Design review of the part built by this model. Coordinates are the model's own, in mm. Face numbers are marked on the shaded views. A direction names the side the tool comes from. Give positions to 0.01 mm unless a question says otherwise; leave off trailing zeros. Loops run counter-clockwise (first coordinate to the right, second up) from the corner with the lowest first, then second, coordinate; pieces in that order, holes last. Notation, with made-up numbers: (64, 7) - (82, 7) arc R26 cw to (82, 31) - close; hole circle Ø10 at (79.25, 67.5). An arc over 180 degrees is marked (long way). Write each question's results on one line, items separated by ' | '.
Autodesk Inventor part; units mm, degrees
ref_plane "YZ Plane" through (0, 0, 0) normal (1, 0, 0) x (0, 1, 0)
ref_plane "XZ Plane" through (0, 0, 0) normal (0, 1, 0) x (-1, 0, 0)
ref_plane "XY Plane" through (0, 0, 0) normal (0, 0, 1) x (1, 0, 0)
sketch "Sketch1" plane through (0, 0, 0) normal (0, 1, 0) x (-1, 0, 0)
  line L0 (-54.2742, 0) -> (84.3226, 0) construction
  line L1 (-6.35, -36.068) -> (57.15, -36.068)
  line L2 (57.15, -36.068) -> (57.15, 36.068)
  line L3 (57.15, 36.068) -> (-6.35, 36.068)
  line L4 (-31.75, 10.668) -> (-31.75, -10.668)
  circle A0 centre (0, 0) radius 17 construction
  circle A1 centre (0, 0) radius 20.81
  line L5 (0, 0) -> (-18.9066, 32.7472) construction
  circle A2 centre (0, 0) radius 3.81 construction
  arc A3 (-6.35, 36.068) -> (-31.75, 10.668) centre (-6.35, 10.668) ccw
  arc A4 (-31.75, -10.668) -> (-6.35, -36.068) centre (-6.35, -10.668) ccw
  circle A5 centre (-12.2465, 21.2116) radius 1.6256 construction
  line L6 (0, 0) -> (31.1733, 53.9938) construction
  circle A6 centre (24.493, 0) radius 1.6256 construction
  circle A7 centre (-12.2465, -21.2116) radius 1.6256 construction
  circle A8 centre (-12.2465, 21.2116) radius 3.175 construction
  point P0 (-31.75, -36.068)
  point P1 (-31.75, 36.068)
  dimension "d0" = 72.136
  dimension "d1" = 88.9
  dimension "d2" = 34
  dimension "d3" = 3.81
  dimension "d4" = 31.75
  dimension "tri_angle" = 120
  dimension "fov_diameter" = 7.62
  dimension "d9" = 25.4
  dimension "d12" = 3.2512
  dimension "mount_radius" = 24.493
  dimension "d14" = 60
  dimension "d25" = 6.35
  dimension "main_aperture_diameter" = 41.62
  dimension "d67" = 2.0574
  dimension "d68" = 10.94
extrude "Extrusion2" add sketch "Sketch1" against normal blind 12.7
sketch "Sketch12" plane through (0, 0, 0) normal (0, 1, 0) x (1, 0, 0)
  line L0 (0, 0) -> (18.9066, -32.7472) construction
  line L1 (12.2465, -21.2116) -> (8.7633, -23.2226) construction
  point P0 (7.2972, -24.0691)
  point P1 (17.1958, -18.3541)
  dimension "d94" = 11.43
sketch "Sketch13" plane through (0, 0, 0) normal (0, 1, 0) x (1, 0, 0)
  line L0 (0, 0) -> (18.9066, -32.7472) construction
  point P0 (12.2465, -21.2116)
hole "Hole4" at (12.2465, 0, 21.2116) direction (0, -1, 0) diameter 6.604 depth 25.4 tip angle 118
sketch "Sketch14" plane through (0, 0, 0) normal (0, 1, 0) x (1, 0, 0)
  line L0 (-112.042, 0) -> (81.9935, 0)
  line L1 (-58.42, 29.1592) -> (-48.26, 29.1592) construction
  line L2 (-58.42, 31.6484) -> (-48.26, 31.6484)
  line L3 (-48.26, 26.67) -> (-58.42, 26.67)
  arc A0 (-58.42, 31.6484) -> (-58.42, 26.67) centre (-58.42, 29.1592) ccw
  arc A1 (-48.26, 26.67) -> (-48.26, 31.6484) centre (-48.26, 29.1592) ccw
  line L4 (-58.42, -31.6484) -> (-48.26, -31.6484)
  line L5 (-48.26, -26.67) -> (-58.42, -26.67)
  arc A2 (-58.42, -26.67) -> (-58.42, -31.6484) centre (-58.42, -29.1592) ccw
  arc A3 (-48.26, -31.6484) -> (-48.26, -26.67) centre (-48.26, -29.1592) ccw
  point P0 (0, 0)
  point P1 (-53.34, 29.1592)
  dimension "d102" = 4.9784
  dimension "d103" = 48.26
  dimension "d104" = 29.1592
  dimension "d105" = 10.16
extrude "Extrusion11" cut sketch "Sketch14" against normal blind 25.4
sketch "Sketch16" plane through (0, 0, 0) normal (0, 1, 0) x (1, 0, 0)
  line L0 (-112.042, 0) -> (81.9935, 0)
  line L1 (0, 50.4952) -> (0, -50.4952)
  arc A0 (-20.81, 0) -> (-20.81, 0) centre (0, 0) ccw
  line L2 (-20.81, 81.7717) -> (-20.81, 0)
  line L3 (0, 0) -> (42.69, 0)
  line L4 (42.69, 0) -> (42.69, 81.7717)
  line L5 (42.69, 81.7717) -> (-20.81, 81.7717)
  line L6 (0, 0) -> (-20.81, 0)
  line L7 (-20.81, 0) -> (-37.279, 0)
  dimension "d112" = 63.5
  dimension "d113" = 81.7717
  dimension "d124" = 0
extrude "Extrusion13" cut sketch "Sketch16" against normal blind 7.9375 contours A0 L1 L0 | L2 L5 L4 L0 A0 | L1 A0 L0 picked at (-13.6994, 1.5436) picked at (7.3346, 11.673)
sketch "Sketch17" plane through (0, -12.7, 0) normal (0, -1, 0) x (1, 0, 0)
  point P0 (0, 0)
  point P1 (7.2972, 24.0691)
  point P2 (17.1958, 18.3541)
hole "Hole6" at (7.2972, -12.7, 24.0691) at (17.1958, -12.7, 18.3541) direction (0, 1, 0) diameter 1.7018 depth 25.4 tip angle 118
sketch "Sketch18" plane through (0, 0, 0) normal (0, 1, 0) x (1, 0, 0)
  line L0 (0, 0) -> (18.9066, -32.7472) construction
  line L1 (7.2972, -24.0691) -> (11.5397, -31.4173) construction
  point P0 (17.1958, -18.3541)
  point P1 (10.4722, -29.5683)
  point P2 (20.3708, -23.8533)
  dimension "d125" = 6.35
hole "Hole7" at (10.4722, 0, 29.5683) at (20.3708, 0, 23.8533) direction (0, -1, 0) diameter 2.159 depth 8.8646 tip angle 118
sketch "Sketch19" plane through (0, 0, 0) normal (0, 1, 0) x (1, 0, 0)
  line L0 (54.2742, 0) -> (-84.3226, 0) construction
  point P0 (0, 0)
  point P1 (0, 0)
  point P2 (-38.1, 19.05)
  point P3 (-38.1, -19.05)
  dimension "d133" = 38.1
  dimension "d134" = 38.1
hole "Hole8" at (-38.1, 0, 19.05) at (-38.1, 0, -19.05) direction (0, -1, 0) diameter 6.7564 depth 19.05 tip angle 118
sketch "Sketch20" plane through (0, 0, 0) normal (0, 1, 0) x (1, 0, 0)
  line L0 (31.75, -10.668) -> (15.3822, -10.668)
  line L1 (15.3822, -10.668) -> (15.3822, -9.652)
  line L2 (15.3822, -9.652) -> (31.75, -9.652)
  line L3 (31.75, -9.652) -> (31.75, -10.668)
  point P0 (0, 0)
  dimension "d142" = 1.016
  dimension "d143" = 16.3678
extrude "Extrusion14" cut sketch "Sketch20" against normal blind 25.4
sketch "Sketch21" plane through (31.75, 0, 0) normal (0, 0, -1) x (-1, 0, 0)
  line L0 (0, -7.9375) -> (0, 0) construction
  line L1 (0, -7.9375) -> (10.94, -7.9375) construction
  line L2 (10.94, 0) -> (10.94, -7.9375) construction
  line L3 (0, 0) -> (10.94, 0) construction
  line L4 (10.94, 0) -> (0, -7.9375) construction
  line L5 (0, 0) -> (25.4, 0) construction
  line L6 (0, -7.9375) -> (10.94, -7.9375) construction
  line L7 (0, 0) -> (10.94, -7.9375) construction
  point P0 (31.75, 0)
  point P1 (5.47, -3.9688)
hole "Hole9" at (26.28, -3.9688, 0) direction (0, 0, 1) diameter 3.2766 depth 10.16
sketch "Sketch22" plane through (31.75, 0, 10.668) normal (0, 0, -1) x (-1, 0, 0)
  point P0 (31.75, 0)
  point P1 (5.47, -3.9688)
hole "Hole10" at (26.28, -3.9688, 10.668) direction (0, 0, 1) diameter 3.302 depth 25.4 tip angle 118
sketch "Sketch23" plane through (0, -12.7, 0) normal (0, -1, 0) x (1, 0, 0)
  line L0 (0, 0) -> (18.9066, 32.7472) construction
  arc A0 (17.8676, 10.668) -> (18.4362, 9.652) centre (0, 0) ccw
  arc A1 (31.75, 10.668) -> (6.35, 36.068) centre (6.35, 10.668) ccw
  circle A2 centre (13.5955, 23.5481) radius 6
  line L1 (6.5804, 20.67) -> (17.5284, 14.3493) construction
  circle A3 centre (12.2465, 21.2116) radius 3.302 construction
  dimension "d160" = 12
extrude "Extrusion15" [suppressed]
equation "\"fov_diameter\" = 2 * d3"
equation "\"d14\" = 0.5 * tri_angle"
equation "\"d15\" = plate_thickness"
equation "\"plate_thickness\" = 12.7"
equation "\"magnet_depth\" = plate_thickness - pin_depth"
equation "\"hole_diameter\" = d2 + fov_diameter"
properties part number "v2_tri_mount"
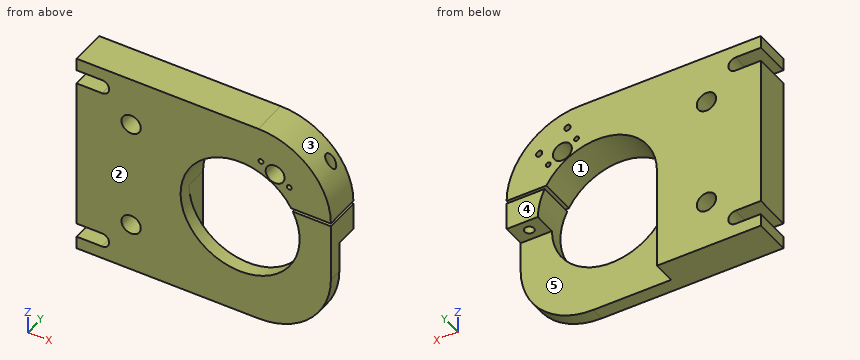
Item 1: Draft analysis for pull direction X (two halves, no side actions). For the marked faces 1, 2 and 3, state which applies: +X half, -X half, draft (parallel to the pull), parting line (faces both ways), or undercut.
Output values:
face 1: undercut | face 2: draft | face 3: +X half
Item 2: Wall thickness on probe 1 along Z at (x, y) = (-38.5, -10); probe 2 along Z at (x, y) = (-48, -5.5); probe 3 along X at (y, z) = (-7.5, 21): over which ranges is each line inside the solid? List them lowest first.
Output values:
probe 1: z = -36.07 to -22.4, -15.7 to 15.7, 22.4 to 36.07 | probe 2: z = -36.07 to -31.63, -26.68 to 26.68, 31.63 to 36.07 | probe 3: x = -57.15 to -40.86, -35.34 to 8.95, 15.54 to 29.55
Item 3: Tool access review of the marked faces 4 and 5: name each direction out of +Z, -Z, +X, -X, +Y, -Y from which nothing blocks a thin tool from reaching the whole face with its end or side.
Output values:
face 4: +Z, -Z, +X, -X, +Y | face 5: -Z, +X, +Y
Item 4: Clearance check with flat-ended pins moving along their axes: P1, Ø3, axis at x = -18.5, z = -10.5, coming from the +Y side; P2, Ø6.5, axis at x = 22, y = -7, coming from the +Z side; P3, Ø1.5, axis at x = 13.5, y = -4.5, coming from the -Z side; P4, Ø5.5, axis at x = -38.1, z = -19.05, coming from the +Y side. State where each tip first meets the part, or that it passes through.
Output values:
P1: stops at y = -7.94 | P2: stops at z = 32.84 | P3: stops at z = 15.17 | P4: passes through
Item 5: We need section A-A on x = -38.1. Give the boundary of the cut face in (y, z), then the cut area to 3 significant figures.
Output values:
outline: (-12.7, -36.07) - (0, -36.07) - (0, -22.43) - (-12.7, -22.43) - close; (-12.7, -15.67) - (0, -15.67) - (0, 15.67) - (-12.7, 15.67) - close; (-12.7, 22.43) - (0, 22.43) - (0, 36.07) - (-12.7, 36.07) - close | area: 745 mm²
Item 6: We need section B-B on z = -19.05. Give the boundary of the cut face in (x, y), then the cut area to 3 significant figures.
Output values:
outline: (-57.15, -12.7) - (-41.48, -12.7) - (-41.48, 0) - (-57.15, 0) - close; (-34.72, -12.7) - (-8.38, -12.7) - (-8.38, -7.94) - (-20.81, -7.94) - (-20.81, 0) - (-34.72, 0) - close; (8.38, -12.7) - (30.33, -12.7) - (30.33, -7.94) - (8.38, -7.94) - close | area: 539 mm²
Item 7: We need section C-C on x = 26.28. Give the boundary of the cut face in (y, z), then the cut area to 3 significant figures.
Output values:
outline: (-12.7, -26.41) - (-7.94, -26.41) - (-7.94, 0) - (-5.61, 0) - (-5.61, 9.65) - (-12.7, 9.65) - close; (-12.7, 10.67) - (-5.62, 10.67) - (-5.62, 26.41) - (-12.7, 26.41) - close; (-2.33, 0) - (0, 0) - (0, 9.65) - (-2.33, 9.65) - close; (-2.32, 10.67) - (0, 10.67) - (0, 26.41) - (-2.32, 26.41) - close | area: 365 mm²
Item 8: We need section D-D on y = -11.5. Give the boundary of the cut face in (x, z).
Output values:
outline: (-57.15, -36.07) - (6.35, -36.07) arc R25.4 ccw to (31.75, -10.67) - (31.75, 9.65) - (18.44, 9.65) arc R20.81 cw (long way) to (17.87, 10.67) - (31.75, 10.67) arc R25.4 ccw to (6.35, 36.07) - (-57.15, 36.07) - (-57.15, 31.65) - (-48.26, 31.65) arc R2.49 cw to (-48.26, 26.67) - (-57.15, 26.67) - (-57.15, -26.67) - (-48.26, -26.67) arc R2.49 cw to (-48.26, -31.65) - (-57.15, -31.65) - close; hole circle Ø6.76 at (-38.1, -19.05); hole circle Ø6.76 at (-38.1, 19.05); hole circle Ø1.7 at (7.3, 24.07); hole circle Ø6.6 at (12.25, 21.21); hole circle Ø1.7 at (17.2, 18.35)
